The model under review builds one solid part; all positions refer to its coordinate system, in mm. Face numbers are marked on the shaded views. A direction names the side the tool comes from. Round coordinates to 2 decimals unless told otherwise and drop trailing zeros. Order: outer loops, then holes, each group sorted by start corner. A loop starts at its lowest first (then second) coordinate and runs counter-clockwise, first axis right, second up.
1) Consider section D-D (y = -4.5). Give the boundary of the cut face in (x, z), then the cut area to 3 significant figures.
2) To check wall thickness, follow L1, parallel to Y at x = -2.55, z = 0; L2, parallel to Z at x = -0.95, y = 0; L3, parallel to Z at x = 1.5, y = 0.5. State the ranges of each line that lie inside material, in increasing order.
3) Machinability: for the marked faces 3, 4, 5, 6 and 7, which of the approach directions +Z, -Z, +X, -X, +Y, -Y give a long, thin tool a straight path to every point of the face, cutting with its end or side? Answer none if there is none.
4) Mouldability with a two-part tool opening along X and no side actions: class the marked faces 1 and 2 as pulls with the +X half, pulls with the -X half, needs draft (parallel to the pull), parting line crosses it, or undercut.
5) Clearance check with flat-ended pins moving along their axes: P1, Ø1, axis at x = -1, z = 1, coming from the -Y side; P2, Ø4, axis at x = -1.5, z = 1.5, coming from the +Y side; P3, Ø4, axis at y = 4, z = 2.5, coming from the +X side. State where each tip first meets the part, or that it passes through.
6) Consider section C-C (x = 8). Give the boundary of the cut face in (y, z), then the cut area to 3 significant figures.
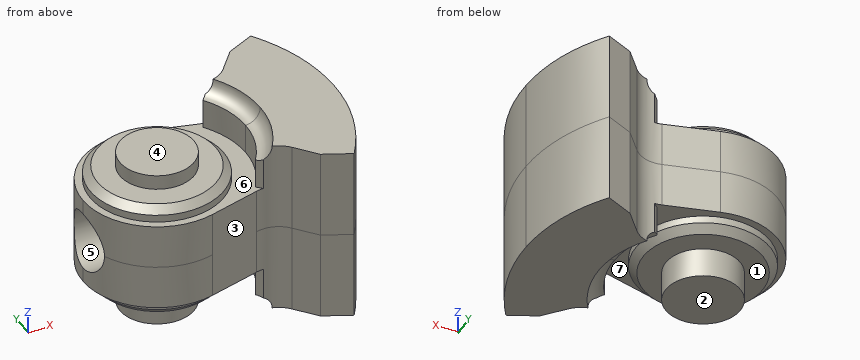
from build123d import *
from build123d import SkipClean  # not in build123d's __all__

# Parameters (mm, degrees)
F1_DEPTH       = 4.7625
F3_DEPTH       = 2.38125
F4_R           = 0.79375
F8_DEPTH       = 25.4
F10_R          = 3.571875
F11_DEPTH      = 3.175
F13_SIZE2      = 0.396875
F13_SIZE       = 0.396875
F12_R          = 1.984375
F15_DEPTH      = 3.96875
F15_DEPTH_BACK = 4.7625
F16_R          = 1.5875
F17_DEPTH      = 25.4


with BuildPart() as f1:
    # F0 (on Top) → F1 (new body)
    with BuildSketch(Plane.XY):
        with BuildLine():
            Line((7.8270786991, 5.4279336804), (6.3629416959, 4.7451953832))
            Line((6.3629416959, 4.7451953832), (5.4090072937, 3.6083406323))
            ThreePointArc((5.4090072937, 3.6083406323), (4.670282197, 3.1147403034), (3.7820365062, 3.0953587134))
            Line((3.7820365062, 3.0953587134), (1.0271880853, 3.8335181231))
            ThreePointArc((1.0271880853, 3.8335181231), (-2.4160219214, 3.1486210693), (-3.96875, 0))
            Line((-3.96875, 0), (9.525, 0))
            ThreePointArc((9.525, 0), (9.0906146549, 2.8436508568), (7.8270786991, 5.4279336804))
        make_face()
    extrude(amount=F1_DEPTH)

    # F2 (on face) → F3 (cut)
    with BuildSketch(Plane.XY.offset(4.7625)):
        with BuildLine():
            Line((3.5700563335, 3.1521586295), (1.0271880853, 3.8335181231))
            ThreePointArc((1.0271880853, 3.8335181231), (-2.4160219214, 3.1486210693), (-3.96875, 0))
            Line((-3.96875, 0), (4.7625, 0))
            ThreePointArc((4.7625, 0), (4.4544247405, 1.6850835234), (3.5700563335, 3.1521586295))
        make_face()
    extrude(amount=-F3_DEPTH, mode=Mode.SUBTRACT)

    # F6: sweep along a path in F5
    with BuildLine(Plane.XY.offset(4.7625)) as f6_path:
        ThreePointArc((4.7625, 0), (4.4544247405, 1.6850835234), (3.5700563335, 3.1521586295))
    # F4 (on Front) → F6 (sweep, cut)
    with BuildSketch(Plane.XZ):
        with Locations((4.7625, 4.7625)):
            Circle(F4_R)
    sweep(path=f6_path.line, mode=Mode.SUBTRACT)

    # F7 (on face) → F8 (cut)
    with BuildSketch(Plane.XY.offset(2.38125)):
        with BuildLine():
            ThreePointArc((3.5700563335, 3.1521586295), (3.7304279124, 2.9606272714), (3.880535973, 2.7609503459))
            Line((3.880535973, 2.7609503459), (4.1611689768, 3.0415833497))
            Line((4.1611689768, 3.0415833497), (4.1606985033, 3.6664465442))
            Line((4.1606985033, 3.6664465442), (2.6852940209, 3.5708183423))
            Line((2.6852940209, 3.5708183423), (3.1285953124, 3.2704477536))
            Line((3.1285953124, 3.2704477536), (3.5700563335, 3.1521586295))
        make_face()
    extrude(amount=F8_DEPTH, mode=Mode.SUBTRACT)

    # F9: F1 across face


with BuildPart() as f1_1:
    add(f1.part, clean=False)
    with SkipClean():  # cleaning this boolean's faces spoils the solid; the shape is the same uncleaned
        add(f1.part.mirror(Plane(origin=(3.9033700373, 0, 1.7817262918), x_dir=(1, 0, 0), z_dir=(0, -1, 0))), clean=False)

    # F10 (on Top) → F11 (join)
    with BuildSketch(Plane.XY):
        Circle(F10_R)
    extrude(amount=F11_DEPTH)

    # F13
    f13_edges = [f1_1.edges().sort_by_distance(p)[0] for p in [
        (-3.571875, 0, 3.175),
    ]]
    chamfer(f13_edges, length=F13_SIZE, length2=F13_SIZE2)

    # F14: F1 across plane


with BuildPart() as f1_2:
    add(f1_1.part, clean=False)
    add(f1_1.part.mirror(Plane.XY), clean=False)

    # F12 (on Top) → F15 (join, two sides)
    with BuildSketch(Plane.XY) as f15_sk:
        Circle(F12_R)
    with SkipClean():  # cleaning this boolean's faces spoils the solid; the shape is the same uncleaned
        extrude(amount=F15_DEPTH)
        extrude(f15_sk.sketch, amount=-F15_DEPTH_BACK)

    # F16 (on Right) → F17 (cut)
    with BuildSketch(Plane.YZ):
        Circle(F16_R)
    with SkipClean():  # cleaning this boolean's faces spoils the solid; the shape is the same uncleaned
        extrude(amount=-F17_DEPTH, mode=Mode.SUBTRACT)


solid = f1_2.part
Answer below:
1. outline: (6.16, -4.76) - (8.39, -4.76) - (8.39, 4.76) - (6.16, 4.76) - close
1. area: 21.3 mm2
2. L1: y = -3.04 to -1.59, 1.59 to 3.04
2. L2: z = -4.76 to -1.59, 1.59 to 3.97
2. L3: z = -4.76 to 3.97
3. face 3: +Z, -Z, -Y
3. face 4: +Z, -X, +Y, -Y
3. face 5: -X
3. face 6: +Z
3. face 7: -Z
4. face 1: undercut
4. face 2: needs draft
5. P1: stops at y = -3.94
5. P2: stops at y = 3.97
5. P3: stops at x = 9.31
6. outline: (-5.17, -4.76) - (5.17, -4.76) - (5.17, 4.76) - (-5.17, 4.76) - close
6. area: 98.5 mm2
